Verification items for the finished model (mm, model axes). A direction names the side the tool comes from. Round coordinates to 2 decimals unless told otherwise and drop trailing zeros. Loops run counter-clockwise (first coordinate to the right, second up) from the corner with the lowest first, then second, coordinate; pieces in that order, holes last. Notation, with made-up numbers: M -32,20 L 19,20 A18 ccw 19,35 Z; hole C 34.25,25.5 d4. An arc over 180 degrees is marked long. Answer as CSV lines item,"result".
```python
from build123d import *

# Parameters (mm, degrees)
BOSS_EXTRUDE1_DEPTH = 3.175
SKETCH4_R           = 2.54
CUT_EXTRUDE12_DEPTH = 3.175


with BuildPart() as part:
    # Sketch2 → Boss-Extrude1 (new body)
    with BuildSketch(Plane(origin=(0, 0, 0), x_dir=(1, 0, 0), z_dir=(0, 1, 0))):
        with BuildLine():
            Line((-12.7, 52.094194642), (-12.7, 197.451116118))
            ThreePointArc((-12.7, 197.451116118), (-11.956051224, 199.247167342), (-10.16, 199.991116118))
            Line((-10.16, 199.991116118), (10.16, 199.991116118))
            ThreePointArc((10.16, 199.991116118), (11.956051224, 199.247167342), (12.7, 197.451116118))
            Line((12.7, 197.451116118), (12.7, 50.8))
            Line((12.7, 50.8), (43.34212974, 28.537189595))
            ThreePointArc((43.34212974, 28.537189595), (44.43776074, 28.083364376), (45.620007447, 28.17640921))
            Line((45.620007447, 28.17640921), (188.881529889, 74.724899563))
            ThreePointArc((188.881529889, 74.724899563), (190.819568924, 74.572372583), (192.082116606, 73.094119178))
            Line((192.082116606, 73.094119178), (198.361341932, 53.768650767))
            ThreePointArc((198.361341932, 53.768650767), (198.208814952, 51.830611732), (196.730561546, 50.568064049))
            Line((196.730561546, 50.568064049), (53.469039104, 4.019573696))
            ThreePointArc((53.469039104, 4.019573696), (52.457891045, 3.399941368), (51.838258718, 2.38879331))
            Line((51.838258718, 2.38879331), (40.533934783, -32.402338363))
            ThreePointArc((40.533934783, -32.402338363), (40.44088995, -33.58458507), (40.894715169, -34.680216069))
            Line((40.894715169, -34.680216069), (126.178179335, -152.062834263))
            ThreePointArc((126.178179335, -152.062834263), (126.632004555, -153.953152345), (125.61625071, -155.610711969))
            Line((125.61625071, -155.610711969), (109.177025385, -167.554508296))
            ThreePointArc((109.177025385, -167.554508296), (107.286707303, -168.008333515), (105.629147678, -166.992579671))
            Line((105.629147678, -166.992579671), (20.345683512, -49.609961478))
            ThreePointArc((20.345683512, -49.609961478), (19.443916216, -48.839779447), (18.290780346, -48.562936018))
            Line((18.290780346, -48.562936018), (-18.290780346, -48.562936018))
            ThreePointArc((-18.290780346, -48.562936018), (-19.443916216, -48.839779447), (-20.345683512, -49.609961478))
            Line((-20.345683512, -49.609961478), (-109.417651575, -172.207007941))
            ThreePointArc((-109.417651575, -172.207007941), (-111.0752112, -173.222761785), (-112.965529282, -172.768936565))
            Line((-112.965529282, -172.768936565), (-129.404754607, -160.825140239))
            ThreePointArc((-129.404754607, -160.825140239), (-130.420508452, -159.167580614), (-129.966683232, -157.277262532))
            Line((-129.966683232, -157.277262532), (-40.894715169, -34.680216069))
            ThreePointArc((-40.894715169, -34.680216069), (-40.44088995, -33.58458507), (-40.533934783, -32.402338363))
            Line((-40.533934783, -32.402338363), (-51.838258718, 2.38879331))
            ThreePointArc((-51.838258718, 2.38879331), (-52.457891045, 3.399941368), (-53.469039104, 4.019573696))
            Line((-53.469039104, 4.019573696), (-197.623627397, 50.858238734))
            ThreePointArc((-197.623627397, 50.858238734), (-199.101880803, 52.120786416), (-199.254407783, 54.058825452))
            Line((-199.254407783, 54.058825452), (-192.975182457, 73.384293863))
            ThreePointArc((-192.975182457, 73.384293863), (-191.712634775, 74.862547268), (-189.77459574, 75.015074248))
            Line((-189.77459574, 75.015074248), (-45.620007447, 28.17640921))
            ThreePointArc((-45.620007447, 28.17640921), (-44.43776074, 28.083364376), (-43.34212974, 28.537189595))
            Line((-43.34212974, 28.537189595), (-13.747025459, 50.039291476))
            ThreePointArc((-13.747025459, 50.039291476), (-12.976843429, 50.941058772), (-12.7, 52.094194642))
        make_face()
    extrude(amount=BOSS_EXTRUDE1_DEPTH)

    # Sketch4 → Cut-Extrude12 (cut)
    with BuildSketch(Plane(origin=(0, 0, 0), x_dir=(1, 0, 0), z_dir=(0, 1, 0))):
        with Locations((0, 63.5)):
            Circle(SKETCH4_R)
        with Locations((60.392088785, 19.622579143)):
            Circle(SKETCH4_R)
        with Locations((37.324363521, -51.372579143)):
            Circle(SKETCH4_R)
        with Locations((-37.324363521, -51.372579143)):
            Circle(SKETCH4_R)
        with Locations((-60.392088785, 19.622579143)):
            Circle(SKETCH4_R)
        with Locations((0, 88.9)):
            Circle(SKETCH4_R)
        with Locations((0, 114.3)):
            Circle(SKETCH4_R)
        with Locations((0, 139.7)):
            Circle(SKETCH4_R)
        with Locations((0, 165.1)):
            Circle(SKETCH4_R)
        with Locations((0, 190.5)):
            Circle(SKETCH4_R)
        with Locations((84.548924299, 27.4716108)):
            Circle(SKETCH4_R)
        with Locations((108.705759813, 35.320642457)):
            Circle(SKETCH4_R)
        with Locations((132.862595326, 43.169674114)):
            Circle(SKETCH4_R)
        with Locations((157.01943084, 51.018705771)):
            Circle(SKETCH4_R)
        with Locations((181.176266354, 58.867737428)):
            Circle(SKETCH4_R)
        with Locations((52.254108929, -71.9216108)):
            Circle(SKETCH4_R)
        with Locations((67.183854337, -92.470642457)):
            Circle(SKETCH4_R)
        with Locations((82.113599745, -113.019674114)):
            Circle(SKETCH4_R)
        with Locations((97.043345153, -133.568705771)):
            Circle(SKETCH4_R)
        with Locations((111.973090562, -154.117737428)):
            Circle(SKETCH4_R)
        with Locations((-52.254108929, -71.9216108)):
            Circle(SKETCH4_R)
        with Locations((-67.183854337, -92.470642457)):
            Circle(SKETCH4_R)
        with Locations((-82.113599745, -113.019674114)):
            Circle(SKETCH4_R)
        with Locations((-97.043345153, -133.568705771)):
            Circle(SKETCH4_R)
        with Locations((-111.973090562, -154.117737428)):
            Circle(SKETCH4_R)
        with Locations((-84.548924299, 27.4716108)):
            Circle(SKETCH4_R)
        with Locations((-108.705759813, 35.320642457)):
            Circle(SKETCH4_R)
        with Locations((-132.862595326, 43.169674114)):
            Circle(SKETCH4_R)
        with Locations((-157.01943084, 51.018705771)):
            Circle(SKETCH4_R)
        with Locations((-181.176266354, 58.867737428)):
            Circle(SKETCH4_R)
    extrude(amount=CUT_EXTRUDE12_DEPTH, mode=Mode.SUBTRACT)


solid = part.part
```
1) Go/stop test with flat-tipped pins: pin 1 (8 mm diameter, centred on x = 0, z = -165.1, fed in from -Y); pin 2 (1 mm diameter, centred on y = 1, z = -150.5, fed in from +X); pin 3 (4 mm diameter, centred on x = 97.04, z = 133.57, fed in from +Y). Record where each tip stops, or that it passes through.
Here are the results:
pin 1,"stops at y = 0"
pin 2,"stops at x = 12.7"
pin 3,"passes through"
2) Draft check along X on faces 1 (the flat face through (-28.75, 1.57, -39.14)), 2 (the flat face through (117.51, 1.57, 161.5)), 3 (the flat face through (0, 0, 0)). Enter one of: +X half, -X half, draft (parallel to the pull), parting line (faces both ways), or undercut.
Here are the results:
face 1,"undercut"
face 2,"+X half"
face 3,"draft"
3) Set-up check for faces 4 (the flat face through (-86.054, 1.565, 96.837)), 5 (the flat face through (27.81, 1.57, -39.82)), 6 (the flat face through (46.265, 1.565, 14.763)), 7 (the flat face through (-64.26, 1.57, 110.05)): record each of +Z, -Z, +X, -X, +Y, -Y from which the full face is reachable in a straight line by a thin tool's end or side.
Here are the results:
face 4,"-X, +Y, -Y"
face 5,"-Z, +Y, -Y"
face 6,"+X, +Y, -Y"
face 7,"+Z, +Y, -Y"
4) Material ranges on probe 1 along Z at (x, y) = (66, 2.55); probe 2 along X at (y, z) = (2.45, -88.9); probe 3 along Z at (x, y) = (111, 0.35), recorded low to high.
Here are the results:
probe 1,"z = -34.8 to -8.09, 69.23 to 90.22, 94.72 to 112.45"
probe 2,"x = -12.7 to -2.54, 2.54 to 12.7"
probe 3,"z = -49.42 to -36.41, -34.23 to -22.71, 131.17 to 151.77, 156.46 to 166.23"
5) Section check B-B (y = 2.65). State how many separate pieces and enclosed holes the cut face has, plus the area to 3 significant figures.
Here are the results:
separate pieces,"1"
enclosed holes,"30"
area,"26,800 mm^2"
6) Section check A-A (z = 103). Record the cut outline in (x, y) (3 decimals).
Here are the results:
outline,"M -90.532,0 L -59.136,0 L -59.136,3.175 L -90.532,3.175 Z; M 59.136,0 L 90.532,0 L 90.532,3.175 L 59.136,3.175 Z"
